Here's how the part is built. I have some questions about the finished solid (model axes, mm). A direction names the side the tool comes from. Round coordinates to 2 decimals unless told otherwise and drop trailing zeros. Loops run counter-clockwise (first coordinate to the right, second up) from the corner with the lowest first, then second, coordinate; pieces in that order, holes last. Notation, with made-up numbers: (37.5, 55.25) - (88.5, 55.25) arc R24 cw to (88.5, 86.25) - close; hole circle Ø2 at (16.25, -36.75). An arc over 180 degrees is marked (long way). Return JSON: item names as keys, results as strings. Group by question number.
```python
from build123d import *

# Parameters (mm, degrees)
CUT_EXTRUDE1_START = -1828.8
CUT_EXTRUDE1_DEPTH = 660.4
SKETCH3_R          = 2.38125
CUT_EXTRUDE3_DEPTH = 50.8
CUT_EXTRUDE4_REACH = 664.838
SKETCH4_R          = 2.413
CUT_EXTRUDE5_REACH = 664.838
SKETCH5_R          = 2.85115
SKETCH6_R          = 2.38125
CUT_EXTRUDE6_DEPTH = 663.837808315


with BuildPart() as part:
    # Cut-Extrude1: read off the stored shape, not the designer's step
    # Cut-Extrude1 outline → Cut-Extrude1 (new body)
    with BuildSketch(Plane.XY.offset(1828.8).offset(CUT_EXTRUDE1_START)):
        with BuildLine():
            Line((0, 50.546), (0, 0.254))
            ThreePointArc((0, 0.254), (0.074394878, 0.074394878), (0.254, 0))
            Line((0.254, 0), (25.146, 0))
            ThreePointArc((25.146, 0), (25.325605122, 0.074394878), (25.4, 0.254))
            Line((25.4, 0.254), (25.4, 50.546))
            ThreePointArc((25.4, 50.546), (25.325605122, 50.725605122), (25.146, 50.8))
            Line((25.146, 50.8), (0.254, 50.8))
            ThreePointArc((0.254, 50.8), (0.074394878, 50.725605122), (0, 50.546))
        make_face()
        with BuildLine():
            ThreePointArc((4.7625, 3.175), (3.639967985, 3.639967985), (3.175, 4.7625))
            Line((3.175, 4.7625), (3.175, 46.0375))
            ThreePointArc((3.175, 46.0375), (3.639967985, 47.160032015), (4.7625, 47.625))
            Line((4.7625, 47.625), (20.6375, 47.625))
            ThreePointArc((20.6375, 47.625), (21.760032015, 47.160032015), (22.225, 46.0375))
            Line((22.225, 46.0375), (22.225, 4.7625))
            ThreePointArc((22.225, 4.7625), (21.760032015, 3.639967985), (20.6375, 3.175))
            Line((20.6375, 3.175), (4.7625, 3.175))
        make_face(mode=Mode.SUBTRACT)
    extrude(amount=CUT_EXTRUDE1_DEPTH)

    # Sketch3 → Cut-Extrude3 (cut)
    with BuildSketch(Plane(origin=(0, 50.8, 0), x_dir=(1, 0, 0), z_dir=(0, 1, 0))):
        with Locations(Location((12.7, -25.4, 0), (0, 0, 270))):
            Circle(SKETCH3_R)
        with Locations(Location((12.7, -12.7, 0), (0, 0, 270))):
            Circle(SKETCH3_R)
        with Locations(Location((12.7, -38.1, 0), (0, 0, 270))):
            Circle(SKETCH3_R)
        with Locations(Location((12.7, -622.3, 0), (0, 0, 270))):
            Circle(SKETCH3_R)
        with Locations(Location((12.7, -635, 0), (0, 0, 270))):
            Circle(SKETCH3_R)
        with Locations(Location((12.7, -647.7, 0), (0, 0, 270))):
            Circle(SKETCH3_R)
        with Locations(Location((12.7, -63.5, 0), (0, 0, 270))):
            Circle(SKETCH3_R)
        with Locations(Location((12.7, -88.9, 0), (0, 0, 270))):
            Circle(SKETCH3_R)
        with Locations(Location((12.7, -596.9, 0), (0, 0, 270))):
            Circle(SKETCH3_R)
        with Locations(Location((12.7, -571.5, 0), (0, 0, 270))):
            Circle(SKETCH3_R)
    extrude(amount=-CUT_EXTRUDE3_DEPTH, mode=Mode.SUBTRACT)

    # Sketch4 → Cut-Extrude4 (cut, up to next)
    with BuildSketch(Plane(origin=(0, 50.8, 0), x_dir=(1, 0, 0), z_dir=(0, 1, 0)), mode=Mode.PRIVATE) as cut_extrude4_sk1:
        with Locations(Location((12.7, -532.289940881, 0), (0, 0, 270))):
            Circle(SKETCH4_R)
    cut_extrude4_tool1 = extrude(cut_extrude4_sk1.sketch, amount=-CUT_EXTRUDE4_REACH, mode=Mode.PRIVATE) & part.part
    # Sketch4 → Cut-Extrude4 (cut, up to next)
    with BuildSketch(Plane(origin=(0, 50.8, 0), x_dir=(1, 0, 0), z_dir=(0, 1, 0)), mode=Mode.PRIVATE) as cut_extrude4_sk2:
        with Locations(Location((12.7, -506.889940881, 0), (0, 0, 270))):
            Circle(SKETCH4_R)
    cut_extrude4_tool2 = extrude(cut_extrude4_sk2.sketch, amount=-CUT_EXTRUDE4_REACH, mode=Mode.PRIVATE) & part.part
    add(cut_extrude4_tool1.solids().sort_by_distance((12.7, 50.8, 532.289941))[0], mode=Mode.SUBTRACT)
    add(cut_extrude4_tool2.solids().sort_by_distance((12.7, 50.8, 506.889941))[0], mode=Mode.SUBTRACT)

    # Sketch5 → Cut-Extrude5 (cut, up to next)
    with BuildSketch(Plane.ZY, mode=Mode.PRIVATE) as cut_extrude5_sk1:
        with Locations((197.92315, 31.33725)):
            Circle(SKETCH5_R)
    cut_extrude5_tool1 = extrude(cut_extrude5_sk1.sketch, amount=-CUT_EXTRUDE5_REACH, mode=Mode.PRIVATE) & part.part
    # Sketch5 → Cut-Extrude5 (cut, up to next)
    with BuildSketch(Plane.ZY, mode=Mode.PRIVATE) as cut_extrude5_sk2:
        with Locations((230.57485, 31.33725)):
            Circle(SKETCH5_R)
    cut_extrude5_tool2 = extrude(cut_extrude5_sk2.sketch, amount=-CUT_EXTRUDE5_REACH, mode=Mode.PRIVATE) & part.part
    # Sketch5 → Cut-Extrude5 (cut, up to next)
    with BuildSketch(Plane.ZY, mode=Mode.PRIVATE) as cut_extrude5_sk3:
        with Locations((230.57485, 6.76275)):
            Circle(SKETCH5_R)
    cut_extrude5_tool3 = extrude(cut_extrude5_sk3.sketch, amount=-CUT_EXTRUDE5_REACH, mode=Mode.PRIVATE) & part.part
    # Sketch5 → Cut-Extrude5 (cut, up to next)
    with BuildSketch(Plane.ZY, mode=Mode.PRIVATE) as cut_extrude5_sk4:
        with Locations((197.92315, 6.76275)):
            Circle(SKETCH5_R)
    cut_extrude5_tool4 = extrude(cut_extrude5_sk4.sketch, amount=-CUT_EXTRUDE5_REACH, mode=Mode.PRIVATE) & part.part
    # Sketch5 → Cut-Extrude5 (cut, up to next)
    with BuildSketch(Plane.ZY, mode=Mode.PRIVATE) as cut_extrude5_sk5:
        with Locations((429.82515, 31.33725)):
            Circle(SKETCH5_R)
    cut_extrude5_tool5 = extrude(cut_extrude5_sk5.sketch, amount=-CUT_EXTRUDE5_REACH, mode=Mode.PRIVATE) & part.part
    # Sketch5 → Cut-Extrude5 (cut, up to next)
    with BuildSketch(Plane.ZY, mode=Mode.PRIVATE) as cut_extrude5_sk6:
        with Locations((462.47685, 31.33725)):
            Circle(SKETCH5_R)
    cut_extrude5_tool6 = extrude(cut_extrude5_sk6.sketch, amount=-CUT_EXTRUDE5_REACH, mode=Mode.PRIVATE) & part.part
    # Sketch5 → Cut-Extrude5 (cut, up to next)
    with BuildSketch(Plane.ZY, mode=Mode.PRIVATE) as cut_extrude5_sk7:
        with Locations((462.47685, 6.76275)):
            Circle(SKETCH5_R)
    cut_extrude5_tool7 = extrude(cut_extrude5_sk7.sketch, amount=-CUT_EXTRUDE5_REACH, mode=Mode.PRIVATE) & part.part
    # Sketch5 → Cut-Extrude5 (cut, up to next)
    with BuildSketch(Plane.ZY, mode=Mode.PRIVATE) as cut_extrude5_sk8:
        with Locations((429.82515, 6.76275)):
            Circle(SKETCH5_R)
    cut_extrude5_tool8 = extrude(cut_extrude5_sk8.sketch, amount=-CUT_EXTRUDE5_REACH, mode=Mode.PRIVATE) & part.part
    add(cut_extrude5_tool1.solids().sort_by_distance((0, 31.33725, 197.92315))[0], mode=Mode.SUBTRACT)
    add(cut_extrude5_tool2.solids().sort_by_distance((0, 31.33725, 230.57485))[0], mode=Mode.SUBTRACT)
    add(cut_extrude5_tool3.solids().sort_by_distance((0, 6.76275, 230.57485))[0], mode=Mode.SUBTRACT)
    add(cut_extrude5_tool4.solids().sort_by_distance((0, 6.76275, 197.92315))[0], mode=Mode.SUBTRACT)
    add(cut_extrude5_tool5.solids().sort_by_distance((0, 31.33725, 429.82515))[0], mode=Mode.SUBTRACT)
    add(cut_extrude5_tool6.solids().sort_by_distance((0, 31.33725, 462.47685))[0], mode=Mode.SUBTRACT)
    add(cut_extrude5_tool7.solids().sort_by_distance((0, 6.76275, 462.47685))[0], mode=Mode.SUBTRACT)
    add(cut_extrude5_tool8.solids().sort_by_distance((0, 6.76275, 429.82515))[0], mode=Mode.SUBTRACT)

    # Sketch6 → Cut-Extrude6 (cut, through all)
    with BuildSketch(Plane.ZY):
        with Locations((214.249, 40.48125)):
            Circle(SKETCH6_R)
        with Locations((446.151, 40.48125)):
            Circle(SKETCH6_R)
    extrude(amount=-CUT_EXTRUDE6_DEPTH, mode=Mode.SUBTRACT)


solid = part.part
```
Q1. Imagine slicing it at A-A, the plane y = 18.5. List the corners of the cut face in (x, z) for me (3 decimals), and give its area (3 significant figures).
Q2. For faces 4 (the flat face through (25.4, 25, 326)), 5 (the flat face through (13, 3.175, 326)), which set-ups out of +Z, -Z, +X, -X, +Y, -Y let a thin tool reach every point of the face, with its end or its side?
Q3. Will these pins go through, and if not, where does the flat tip stop? pin 1 Ø3 at (x, z) = (12.7, 596.9) entering from +Y; pin 2 Ø5.5 at (x, z) = (12.7, 647.7) entering from -Y; pin 3 Ø4.5 at (y, z) = (31.34, 230.57) entering from -X (3 decimals).
Q4. Please list where these lines run through material, in increasing order: line 1 (X direction, y = 36.5, z = 210) (3 decimals); line 2 (Y direction, x = 12.5, z = 551) (3 decimals); line 3 (Z direction, x = 2, y = 39).
Q5. If we mould it in two halves opening along Y, with no side actions, what happens to faces 1 (the flat face through (2, 24, 660.4)), 2 (the flat face through (13, 50.8, 326)), 3 (the flat face through (22.225, 26, 326))? For each: +Y half, -Y half, draft (parallel to the pull), parting line (faces both ways), or undercut.
Output values:
{
 "1": {"outline": "(0, 0) - (3.175, 0) - (3.175, 660.4) - (0, 660.4) - close; (22.225, 0) - (25.4, 0) - (25.4, 660.4) - (22.225, 660.4) - close", "area": "4,190 mm^2"},
 "2": {"face 4": "+Z, -Z, +X, +Y, -Y", "face 5": "+Z, -Z"},
 "3": {"pin 1": "passes through", "pin 2": "stops at y = 0", "pin 3": "stops at x = 22.225"},
 "4": {"line 1": "x = 0 to 3.175, 22.225 to 25.4", "line 2": "y = 0 to 3.175, 47.625 to 50.8", "line 3": "z = 0 to 212.38, 216.11 to 444.29, 448.02 to 660.4"},
 "5": {"face 1": "draft", "face 2": "+Y half", "face 3": "undercut"}
}
